from build123d import *

# Parameters (mm, degrees)
CORTE_EXTRUS_O1_DEPTH = 0.5


with BuildPart() as part:
    # Esboço1 → Revolução1 (revolve)
    with BuildSketch(Plane.XY, mode=Mode.PRIVATE) as revolu_o1_sk:
        with BuildLine():
            Line((0, 32), (2, 32))
            ThreePointArc((2, 32), (2.353553391, 31.853553391), (2.5, 31.5))
            Line((2.5, 31.5), (2.5, 30))
            Line((2.5, 30), (1.5, 30))
            Line((1.5, 30), (1.5, 0))
            Line((1.5, 0), (0, 0))
            Line((0, 0), (0, 32))
        make_face()
    revolve(revolu_o1_sk.sketch.rotate(Axis((0, 32, 0), (0, -1, 0)), 180), axis=Axis((0, 32, 0), (0, -1, 0)))

    # Esboço2 → Corte-extrusão1 (cut)
    with BuildSketch(Plane(origin=(0, 32, 0), x_dir=(1, 0, 0), z_dir=(0, 1, 0))):
        Polygon((-1.236731601, 1.156201078), (-0.281827121, 0.023947316), (-1.414080883, -0.930957165), (-1.156201078, -1.236731601), (-0.023947316, -0.281827121), (0.930957165, -1.414080883), (1.236731601, -1.156201078), (0.281827121, -0.023947316), (1.414080883, 0.930957165), (1.156201078, 1.236731601), (0.023947316, 0.281827121), (-0.930957165, 1.414080883), align=None)
    extrude(amount=-CORTE_EXTRUS_O1_DEPTH, mode=Mode.SUBTRACT)


solid = part.part
Build history of the part. All positions in model axes, mm. A direction names the side the tool comes from. Coordinates: 2 decimals unless noted, no trailing zeros. Order: outer loops, then holes, each group sorted by start corner. A loop starts at its lowest first (then second) coordinate and runs counter-clockwise, first axis right, second up. Notation, with made-up numbers: (-8.75, -18) - (38.25, -18) arc R28 ccw to (38.25, 0) - close; hole circle Ø3 at (46.5, 10). An arc over 180 degrees is marked (long way). Write item = value, one per line. Start each with the question number.
1) Flat gauge pins, fed straight in: pin 1 Ø3 at (x, y) = (-1, 16.5) entering from -Z; pin 2 Ø1.5 at (y, z) = (12.5, 1) entering from -X. Where does each tip first touch, or does it go through?
2) 3-axis set-ups, long thin cutter, end or side, ignore diameter. For faces 1 (the face through (0.447, 31.754, 0.84)), 2 (the face through (-1.43, 14.79, -0.45)), 3 (the face through (0, 0, 0)): which of +Z, -Z, +X, -X, +Y, -Y reach the whole face in a straight line?
3) Saw through at A-A on y = 27. Write the cut outline in (x, z).
4) Wall check: line 1 along Y through (x, z) = (0.9, -1.3); line 2 along Z through (x, y) = (0, 18.5). Give the ranges that are in metal, low to high. Write a range as from..to.
From the geometry:
q1.pin_1 = -1.5
q1.pin_2 = -1.48
q2.face_1 = +Y
q2.face_2 = -Y
q2.face_3 = +Z, -Z, +X, -X, -Y
q3.outline = circle Ø3 at (0, 0)
q4.line_1 = 30..32
q4.line_2 = -1.5..1.5
